Model file for the job. Use its own axes, mm. Face numbers are marked on the shaded views. Coordinates: 2 decimals unless noted, no trailing zeros. Loops run counter-clockwise (first coordinate to the right, second up) from the corner with the lowest first, then second, coordinate; pieces in that order, holes last. Notation, with made-up numbers: M -23,-19.5 L 26,-19.5 A25 ccw 26,12.5 Z; hole C 76.5,-11.5 d9. An arc over 180 degrees is marked long. Write item = value, one per line. Start each with the question number.
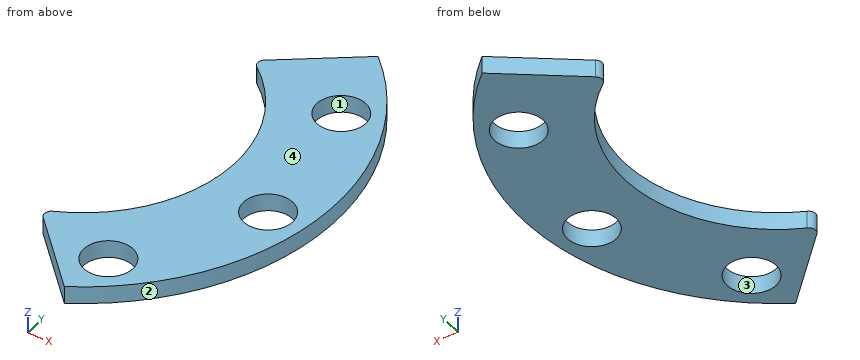
from build123d import *

# Parameters (mm, degrees)
SKETCH6_R           = 6.5
SKETCH6_R_2         = 4.445
BOSS_EXTRUDE3_DEPTH = 3.175


with BuildPart() as part:
    # Sketch6 → Boss-Extrude3 (new body)
    # profile 1 of 4: a face of its own
    with BuildSketch(Plane.XY):
        with BuildLine():
            Line((16.779877408, 23.796523986), (30.381235635, 34.235995151))
            ThreePointArc((30.381235635, 34.235995151), (45.571708019, -4.282787757), (23.47067629, -39.296948955))
            Line((23.47067629, -39.296948955), (11.181031284, -27.004389661))
            ThreePointArc((11.181031284, -27.004389661), (10.828800328, -25.884001858), (11.545866958, -24.953866964))
            ThreePointArc((11.545866958, -24.953866964), (27.324797823, -3.059075709), (16.778161303, 21.782925045))
            ThreePointArc((16.778161303, 21.782925045), (16.283134573, 22.790147137), (16.779877408, 23.796523986))
        make_face()
        with Locations((33.774990729, 19.499999989)):
            Circle(SKETCH6_R, mode=Mode.SUBTRACT)
        with Locations((25.068716764, -29.875733265)):
            Circle(SKETCH6_R, mode=Mode.SUBTRACT)
        with Locations((38.407502346, -6.772278925)):
            Circle(SKETCH6_R, mode=Mode.SUBTRACT)
    # profile 2 of 4: a face of its own
    with BuildSketch(Plane.XY):
        with Locations((25.068716764, -29.875733265)):
            Circle(SKETCH6_R)
        with Locations((25.068716764, -29.875733265)):
            Circle(SKETCH6_R_2, mode=Mode.SUBTRACT)
    # profile 3 of 4: a face of its own
    with BuildSketch(Plane.XY):
        with Locations((38.407502346, -6.772278925)):
            Circle(SKETCH6_R)
        with Locations((38.407502346, -6.772278925)):
            Circle(SKETCH6_R_2, mode=Mode.SUBTRACT)
    # profile 4 of 4: a face of its own
    with BuildSketch(Plane.XY):
        with Locations((33.774990729, 19.499999989)):
            Circle(SKETCH6_R)
        with Locations((33.774990729, 19.499999989)):
            Circle(SKETCH6_R_2, mode=Mode.SUBTRACT)
    extrude(amount=BOSS_EXTRUDE3_DEPTH)


solid = part.part
Item 1: Pull direction X, two halves, no side cores. Call the marked faces 1, 2, 3 and 4: +X half, -X half, draft (parallel to the pull), parting line (faces both ways), or undercut.
Item 2: Pin check, flat tips, straight feed: pin 1 Ø5.5 at (x, y) = (38.41, -6.77) entering from -Z; pin 2 Ø1.5 at (y, z) = (-10.5, 1) entering from +X; pin 3 Ø1 at (x, z) = (41.5, 2) entering from +Y; pin 4 Ø1.5 at (y, z) = (20.5, 2.5) entering from -X. Stop position of each tip, or through.
Item 3: Cut at C-C (y = -5). Give the cut face in (x, z) (3 decimals), plus the area to 3 significant figures.
Item 4: Cut at B-B (z = 1.9). Give the cut face in (x, y) (1 decimal), plus the area to 3 significant figures.
Item 5: Probe L1, parallel to Y at x = 25, z = 1.9; L2, parallel to Y at x = 32.5, z = 1.8; L3, parallel to X at y = 0.5, z = 0.7. List the from-to ranges inside material, lowest first.
Item 6: Cut at D-D (x = 13). Give the cut face in (y, z) (3 decimals), plus the area to 3 significant figures.
Item 7: Cut at A-A (y = 19.5). Give the cut face in (x, z) (3 decimals).
Reported:
q1.face_1 = undercut
q1.face_2 = +X half
q1.face_3 = undercut
q1.face_4 = draft
q2.pin_1 = through
q2.pin_2 = 44.72
q2.pin_3 = 20.35
q2.pin_4 = 17.45
q3.outline = M 27.037,0 L 34.331,0 L 34.331,3.175 L 27.037,3.175 Z; M 42.484,0 L 45.499,0 L 45.499,3.175 L 42.484,3.175 Z
q3.area = 32.7 mm^2
q4.outline = M 11.2,-27 L 23.5,-39.3 A45.8 ccw 30.4,34.2 L 16.8,23.8 A1.3 ccw 16.8,21.8 A27.5 cw 11.5,-25 A1.3 ccw Z; hole C 25.1,-29.9 d8.9; hole C 33.8,19.5 d8.9; hole C 38.4,-6.8 d8.9
q4.area = 1,140 mm^2
q5.L1 = -38.34 to -34.32, -25.43 to -11.45, 11.45 to 30.11
q5.L2 = -32.23 to 15.24, 23.76 to 32.23
q5.L3 = 27.49 to 45.77
q6.outline = M -28.824,0 L -24.228,0 L -24.228,3.175 L -28.824,3.175 Z
q6.area = 14.6 mm^2
q7.outline = M 19.384,0 L 29.33,0 L 29.33,3.175 L 19.384,3.175 Z; M 38.22,0 L 41.411,0 L 41.411,3.175 L 38.22,3.175 Z
